Could you check a few things on this model? Use its own coordinates, in mm. A direction names the side the tool comes from. Coordinates: 2 decimals unless noted, no trailing zeros. Order: outer loops, then holes, each group sorted by start corner. A loop starts at its lowest first (then second) coordinate and runs counter-clockwise, first axis right, second up. Notation, with made-up numbers: (84, 15.5) -> (131, 15.5) arc R13 ccw to (131, 30.5) -> close; hole circle Ø9 at (68, 77). An arc over 180 degrees is marked (long way). Use a Markdown table: item, result. Add a question column.
1) If we section it at A-A (z = 17): Write out the boundary of the cut face in (x, y).
2) Which directions (+Z, -Z, +X, -X, +Y, -Y) give clear straight access to the entire face, cutting with the end or side of a thin tool? Please do faces 1 (the flat face through (4.7, -9, 12)), 2 (the flat face through (-5, 0, 12)), 3 (the flat face through (-5, -9, 12)), 4 (the flat face through (5, -3.729, 12)).
3) If we section it at B-B (x = 0): Write out the boundary of the cut face in (y, z).
4) If we section it at C-C (y = 1.5): Write out the boundary of the cut face in (x, z).
5) Will these pins go through, and if not, where does the flat tip stop? pin 1 Ø1 at (x, z) = (5, 8) entering from -Y; pin 2 Ø6 at (x, z) = (3.5, 9.5) entering from -Y; pin 3 Ø8 at (x, y) = (0, -2.5) entering from -Z; pin 4 Ø5.5 at (y, z) = (-0.5, 7.5) entering from +X.
6) If we section it at D-D (x = 1.75): Write out the boundary of the cut face in (y, z).
7) If I drill on L1, parallel to Z at x = 0, y = -0.5; L2, parallel to X at y = 0.75, z = 22.75; L3, parallel to Y at x = 5.5, z = 2.75, over which ranges is the centre line in solid material (lowest first)? Write a range as [from, to].
```python
from build123d import *

# Parameters (mm, degrees)
F0_W     = 9.7
F0_H     = 7.1
F0_H_2   = 4.7
F0_W_2   = 2.5
F0_H_3   = 1.2
F1_DEPTH = 25
F2_R     = 1
F3_R     = 1
F4_DEPTH = 17.5645790518
F5_R     = 1
F6_DEPTH = 22.29565


with BuildPart() as f1:
    # F0 (on Top) → F1 (new body)
    with BuildSketch(Plane.XY):
        with Locations((-0.15, -0.179021287)):
            Rectangle(F0_W, F0_H)
        with Locations((-0.15, -6.079021287)):
            Rectangle(F0_W, F0_H_2)
        with Locations((-6.25, -6.079021287)):
            Rectangle(F0_W_2, F0_H_2)
        with Locations((5.95, -6.079021287)):
            Rectangle(F0_W_2, F0_H_2)
        with Locations((-0.15, -9.029021287)):
            Rectangle(F0_W, F0_H_3)
        Polygon((4.7, -9.629021287), (-5, -9.629021287), (0, -14.629021287), align=None)
    extrude(amount=F1_DEPTH)

    # F2
    f2_edges = [f1.edges().sort_by_distance(p)[0] for p in [
        (-7.5, -3.729021, 12.5),
        (-7.5, -8.429021, 12.5),
        (7.2, -3.729021, 12.5),
        (7.2, -8.429021, 12.5),
        (0, -14.629021, 12.5),
    ]]
    fillet(f2_edges, radius=F2_R)

    # F3 (on face) → F4 (cut, through all)
    with BuildSketch(Plane(origin=(0, 3.370978713, 0), x_dir=(-1, 0, 0), z_dir=(0, 1, 0))):
        with Locations((0, 12.7671947703)):
            Circle(F3_R)
    extrude(amount=-F4_DEPTH, mode=Mode.SUBTRACT)

    # F5 (on face) → F6 (cut)
    with BuildSketch(Plane(origin=(0, 3.370978713, 0), x_dir=(-1, 0, 0), z_dir=(0, 1, 0))):
        with Locations((0, 18.7855240438)):
            Circle(F5_R)
    extrude(amount=F6_DEPTH, mode=Mode.SUBTRACT)


solid = f1.part
```
Answer sheet:
| question | item | result |
|---|---|---|
| 1 | outline | (-7.5, -7.43) arc R1 ccw to (-6.5, -8.43) -> (-5, -8.43) -> (-5, -9.63) -> (-0.73, -13.9) arc R1 ccw to (0.71, -13.88) -> (4.7, -9.63) -> (4.7, -8.43) -> (6.2, -8.43) arc R1 ccw to (7.2, -7.43) -> (7.2, -4.73) arc R1 ccw to (6.2, -3.73) -> (4.7, -3.73) -> (4.7, 3.37) -> (-5, 3.37) -> (-5, -3.73) -> (-6.5, -3.73) arc R1 ccw to (-7.5, -4.73) -> close |
| 2 | face 1 | +Z, -Z, +X, -Y |
| 2 | face 2 | +Z, -Z, -X, +Y |
| 2 | face 3 | +Z, -Z, -X, -Y |
| 2 | face 4 | +Z, -Z, +X, +Y |
| 3 | outline | (-14.19, 0) -> (3.37, 0) -> (3.37, 11.77) -> (-14.19, 11.77) -> close; (-14.19, 13.77) -> (3.37, 13.77) -> (3.37, 25) -> (-14.19, 25) -> close |
| 4 | outline | (-5, 0) -> (4.7, 0) -> (4.7, 25) -> (-5, 25) -> close; hole circle Ø2 at (0, 12.77) |
| 5 | pin 1 | y = -9.84 |
| 5 | pin 2 | y = -14.05 |
| 5 | pin 3 | z = 0 |
| 5 | pin 4 | x = 4.7 |
| 6 | outline | (-12.77, 0) -> (3.37, 0) -> (3.37, 25) -> (-12.77, 25) -> close |
| 7 | L1 | [0, 11.77], [13.77, 25] |
| 7 | L2 | [-5, 4.7] |
| 7 | L3 | [-8.43, -3.73] |
